Could you check a few things on this model? Use its own coordinates, in mm. Face numbers are marked on the shaded views. Coordinates: 2 decimals unless noted, no trailing zeros. Loops run counter-clockwise (first coordinate to the right, second up) from the corner with the lowest first, then second, coordinate; pieces in that order, holes last. Notation, with made-up numbers: (-12.5, 57) -> (-3.5, 57) arc R26 cw to (-3.5, 73) -> close; hole circle Ø6 at (33.25, -38). An arc over 180 degrees is marked (long way). One line per question, with ' | ' between items. Start each with the question number.
(1) Suppose I cut it at C-C (z = 4.25). Please give me the cut outline in (x, y), plus the area to 3 significant figures.
(2) If I drill on line 1 along X through (y, z) = (0.1, -8.5); line 2 along X through (y, z) = (0.1, 0.75); line 3 along X through (y, z) = (0.45, -3), over which ranges is the centre line in solid material (lowest first)?
(3) If we mould it in two halves opening along X, with no side actions, what happens to the marked faces 1 and 2? For each: pulls with the +X half, pulls with the -X half, needs draft (parallel to the pull), parting line crosses it, or undercut.
(4) Suppose I cut it at B-B (x = -0.5). Please give me the cut outline in (y, z).
(5) Suppose I cut it at A-A (z = -3). Please give me the cut outline in (x, y), plus the area to 3 significant figures.
(6) I'm going to push flat-ended pins straight in: pin 1 Ø2 at (x, z) = (-9, 8.5) entering from +Y; pin 2 Ø1.3 at (x, z) = (-9, 5.53) entering from +Y. Where does each tip first touch, or does it pass through?
(7) Suppose I cut it at D-D (y = 0.2). Give the number of separate pieces and of enclosed holes in the cut face, plus the area to 3 significant figures.
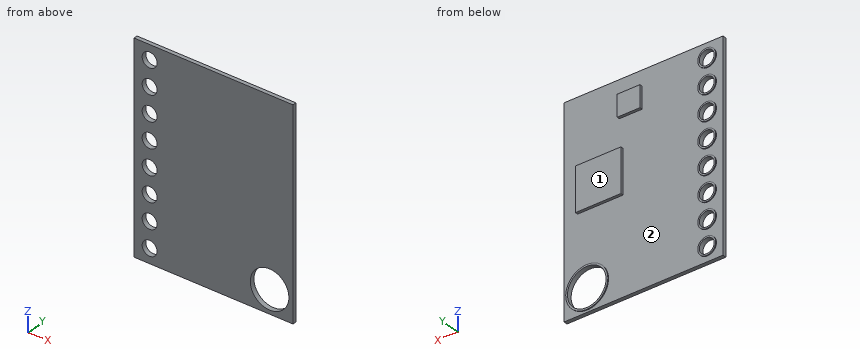
```python
from build123d import *

# Parameters (mm, degrees)
SKETCH1_W           = 17
SKETCH1_H           = 22
SKETCH1_R           = 2.066566425
SKETCH1_R_2         = 0.8
BOSS_EXTRUDE2_DEPTH = 0.4
SKETCH3_R           = 2.253615782
SKETCH3_R_2         = 2.066566425
SKETCH3_R_3         = 0.962856641
SKETCH3_R_4         = 0.8
BOSS_EXTRUDE3_DEPTH = 0.1
SKETCH4_W           = 2.432070337
SKETCH4_H           = 2.310466819
SKETCH4_W_2         = 4.864140673
SKETCH4_H_2         = 4.681735398
BOSS_EXTRUDE4_DEPTH = 0.3


with BuildPart() as part:
    # Sketch1 → Boss-Extrude2 (new body)
    with BuildSketch(Plane(origin=(0, 0, 0), x_dir=(1, 0, 0), z_dir=(0, 1, 0))):
        with Locations((-2.156716418, -1.485074627)):
            Rectangle(SKETCH1_W, SKETCH1_H)
        with Locations(Location((3.843283582, 7.034200162, 0), (0, 0, 270))):
            Circle(SKETCH1_R, mode=Mode.SUBTRACT)
        with Locations(Location((-8.998366841, 7.966442948, 0), (0, 0, 270))):
            Circle(SKETCH1_R_2, mode=Mode.SUBTRACT)
        with Locations(Location((-8.998366841, 5.266442948, 0), (0, 0, 270))):
            Circle(SKETCH1_R_2, mode=Mode.SUBTRACT)
        with Locations(Location((-8.998366841, 2.566442948, 0), (0, 0, 270))):
            Circle(SKETCH1_R_2, mode=Mode.SUBTRACT)
        with Locations(Location((-8.998366841, -0.133557052, 0), (0, 0, 270))):
            Circle(SKETCH1_R_2, mode=Mode.SUBTRACT)
        with Locations(Location((-8.998366841, -2.833557052, 0), (0, 0, 270))):
            Circle(SKETCH1_R_2, mode=Mode.SUBTRACT)
        with Locations(Location((-8.998366841, -5.533557052, 0), (0, 0, 270))):
            Circle(SKETCH1_R_2, mode=Mode.SUBTRACT)
        with Locations(Location((-8.998366841, -8.233557052, 0), (0, 0, 270))):
            Circle(SKETCH1_R_2, mode=Mode.SUBTRACT)
        with Locations(Location((-8.998366841, -10.933557052, 0), (0, 0, 270))):
            Circle(SKETCH1_R_2, mode=Mode.SUBTRACT)
    extrude(amount=BOSS_EXTRUDE2_DEPTH)

    # Sketch3 → Boss-Extrude3 (add)
    # profile 1 of 9: a face of its own
    with BuildSketch(Plane(origin=(0, 0.4, 0), x_dir=(1, 0, 0), z_dir=(0, 1, 0))):
        with Locations(Location((3.843283582, 7.034200162, 0), (0, 0, 270))):
            Circle(SKETCH3_R)
        with Locations(Location((3.843283582, 7.034200162, 0), (0, 0, 270))):
            Circle(SKETCH3_R_2, mode=Mode.SUBTRACT)
    # profile 2 of 9: a face of its own
    with BuildSketch(Plane(origin=(0, 0.4, 0), x_dir=(1, 0, 0), z_dir=(0, 1, 0))):
        with Locations(Location((-8.998366841, 7.966442948, 0), (0, 0, 270))):
            Circle(SKETCH3_R_3)
        with Locations(Location((-8.998366841, 7.966442948, 0), (0, 0, 270))):
            Circle(SKETCH3_R_4, mode=Mode.SUBTRACT)
    # profile 3 of 9: a face of its own
    with BuildSketch(Plane(origin=(0, 0.4, 0), x_dir=(1, 0, 0), z_dir=(0, 1, 0))):
        with Locations(Location((-8.998366841, 5.266442948, 0), (0, 0, 270))):
            Circle(SKETCH3_R_3)
        with Locations(Location((-8.998366841, 5.266442948, 0), (0, 0, 270))):
            Circle(SKETCH3_R_4, mode=Mode.SUBTRACT)
    # profile 4 of 9: a face of its own
    with BuildSketch(Plane(origin=(0, 0.4, 0), x_dir=(1, 0, 0), z_dir=(0, 1, 0))):
        with Locations(Location((-8.998366841, 2.566442948, 0), (0, 0, 270))):
            Circle(SKETCH3_R_3)
        with Locations(Location((-8.998366841, 2.566442948, 0), (0, 0, 270))):
            Circle(SKETCH3_R_4, mode=Mode.SUBTRACT)
    # profile 5 of 9: a face of its own
    with BuildSketch(Plane(origin=(0, 0.4, 0), x_dir=(1, 0, 0), z_dir=(0, 1, 0))):
        with Locations(Location((-8.998366841, -0.133557052, 0), (0, 0, 270))):
            Circle(SKETCH3_R_3)
        with Locations(Location((-8.998366841, -0.133557052, 0), (0, 0, 270))):
            Circle(SKETCH3_R_4, mode=Mode.SUBTRACT)
    # profile 6 of 9: a face of its own
    with BuildSketch(Plane(origin=(0, 0.4, 0), x_dir=(1, 0, 0), z_dir=(0, 1, 0))):
        with Locations(Location((-8.998366841, -2.833557052, 0), (0, 0, 270))):
            Circle(SKETCH3_R_3)
        with Locations(Location((-8.998366841, -2.833557052, 0), (0, 0, 270))):
            Circle(SKETCH3_R_4, mode=Mode.SUBTRACT)
    # profile 7 of 9: a face of its own
    with BuildSketch(Plane(origin=(0, 0.4, 0), x_dir=(1, 0, 0), z_dir=(0, 1, 0))):
        with Locations(Location((-8.998366841, -5.533557052, 0), (0, 0, 270))):
            Circle(SKETCH3_R_3)
        with Locations(Location((-8.998366841, -5.533557052, 0), (0, 0, 270))):
            Circle(SKETCH3_R_4, mode=Mode.SUBTRACT)
    # profile 8 of 9: a face of its own
    with BuildSketch(Plane(origin=(0, 0.4, 0), x_dir=(1, 0, 0), z_dir=(0, 1, 0))):
        with Locations(Location((-8.998366841, -8.233557052, 0), (0, 0, 270))):
            Circle(SKETCH3_R_3)
        with Locations(Location((-8.998366841, -8.233557052, 0), (0, 0, 270))):
            Circle(SKETCH3_R_4, mode=Mode.SUBTRACT)
    # profile 9 of 9: a face of its own
    with BuildSketch(Plane(origin=(0, 0.4, 0), x_dir=(1, 0, 0), z_dir=(0, 1, 0))):
        with Locations(Location((-8.998366841, -10.933557052, 0), (0, 0, 270))):
            Circle(SKETCH3_R_3)
        with Locations(Location((-8.998366841, -10.933557052, 0), (0, 0, 270))):
            Circle(SKETCH3_R_4, mode=Mode.SUBTRACT)
    extrude(amount=BOSS_EXTRUDE3_DEPTH)

    # Sketch4 → Boss-Extrude4 (add)
    with BuildSketch(Plane(origin=(0, 0.4, 0), x_dir=(1, 0, 0), z_dir=(0, 1, 0))):
        with Locations((-0.788676854, -9.708512452)):
            Rectangle(SKETCH4_W, SKETCH4_H)
        with Locations((2.464217222, -3.081120785)):
            Rectangle(SKETCH4_W_2, SKETCH4_H_2)
    extrude(amount=BOSS_EXTRUDE4_DEPTH)


solid = part.part
```
Checks:
1) outline: (-10.66, 0) -> (6.34, 0) -> (6.34, 0.4) -> (4.9, 0.4) -> (4.9, 0.7) -> (0.03, 0.7) -> (0.03, 0.4) -> (-10.66, 0.4) -> close | area: 8.26 mm^2
2) line 1: x = -10.66 to -9.59, -8.4 to 2.39, 5.3 to 6.34 | line 2: x = -10.66 to -9.51, -8.49 to 6.34 | line 3: x = -9.86 to -9.67, -8.33 to -8.14
3) face 1: needs draft | face 2: undercut
4) outline: (0, -9.51) -> (0.4, -9.51) -> (0.4, 8.55) -> (0.7, 8.55) -> (0.7, 10.86) -> (0.4, 10.86) -> (0.4, 12.49) -> (0, 12.49) -> close
5) outline: (-10.66, 0) -> (-9.67, 0) -> (-9.67, 0.5) -> (-9.86, 0.5) -> (-9.86, 0.4) -> (-10.66, 0.4) -> close; (-8.33, 0) -> (6.34, 0) -> (6.34, 0.4) -> (-8.14, 0.4) -> (-8.14, 0.5) -> (-8.33, 0.5) -> close | area: 6.30 mm^2
6) pin 1: stops at y = 0.5 | pin 2: passes through
7) separate pieces: 1 | enclosed holes: 9 | area: 344 mm^2
